Solid Edge part; units mm, degrees
sketch "Sketch1" plane through (0, 0, 0) normal (0, 0, 1) x (1, 0, 0)
  circle A0 centre (0, 0) radius 1.5
extrude "Protrusion1" add sketch "Sketch1" along normal blind 30
chamfer "Chaflán_1" distance 0.6 angle 45 1 edges at (-1.5, 0, 0)
sketch "Sketch2" plane through (0, 0, 30) normal (0, 0, 1) x (1, 0, 0)
  circle A0 centre (0, 0) radius 2.7
extrude "ProtrusiónExtruida_3" add sketch "Sketch2" along normal blind 2
sketch "Sketch3" plane through (0, 0, 32) normal (0, 0, 1) x (0, 1, 0)
  line L0 (0.5, -3.2084) -> (-0.5, -3.2084)
  line L1 (-0.5, -3.2084) -> (-0.5, 3.2084)
  line L2 (-0.5, 3.2084) -> (0.5, 3.2084)
  line L3 (0.5, 3.2084) -> (0.5, -3.2084)
extrude "VaciadoExtruido_5" cut sketch "Sketch3" against normal blind 1.148
properties material "Acero inoxidable, 303"
Here's how the part is built. I have some questions about the finished solid (model axes, mm). A direction names the side the tool comes from. Coordinates: 2 decimals unless noted, no trailing zeros. Order: outer loops, then holes, each group sorted by start corner. A loop starts at its lowest first (then second) coordinate and runs counter-clockwise, first axis right, second up.
1) I need wall thicknesses on line 1 (Y direction, x = -1.2, z = 21.5); line 2 (Z direction, x = 1.1, y = -1.25); line 3 (X direction, y = -0.55, z = 23). Which ranges of each line are inside material? Lowest first, please.
2) Imagine slicing it at B-B on x = 0. List the corners of the cut face in (y, z) for me.
3) We'd pull the mould along Y, two halves only. Please class faces 4 (the face through (1.2, -1.2, 30)), 5 (the face through (2.575, -0.811, 30.986)), 6 (the face through (0, 0.5, 31.4)): +Y half, -Y half, draft (parallel to the pull), parting line (faces both ways), or undercut.
4) Imagine slicing it at D-D on x = -2.3. List the corners of the cut face in (y, z) for me.
5) Imagine slicing it at A-A on y = 0. List the corners of the cut face in (x, z) for me.
6) Imagine slicing it at C-C on z = 6. List the corners of the cut face in (x, y) for me, and give its area (3 significant figures).
7) Will these pins go through, and if not, where does the flat tip stop? pin 1 (1 mm diameter, centred on x = -1, z = 10.5, fed in from -Y); pin 2 (1.5 mm diameter, centred on x = -1, z = 4.5, fed in from -Y); pin 3 (1 mm diameter, centred on x = -1, z = 15.5, fed in from +Y).
8) Which directions (+Z, -Z, +X, -X, +Y, -Y) give clear straight access to the entire face, cutting with the end or side of a thin tool? Please do faces 1 (the face through (0, -0.5, 31.4)), 2 (the face through (-1.5, -0.07, 15.09)), 3 (the face through (0, -1, 32)).
Response values:
1. line 1: y = -0.9 to 0.9
1. line 2: z = 30 to 32
1. line 3: x = -1.4 to 1.4
2. outline: (-2.7, 30) - (-1.5, 30) - (-1.5, 0.6) - (-0.9, 0) - (0.9, 0) - (1.5, 0.6) - (1.5, 30) - (2.7, 30) - (2.7, 32) - (0.5, 32) - (0.5, 30.85) - (-0.5, 30.85) - (-0.5, 32) - (-2.7, 32) - close
3. face 4: draft
3. face 5: parting line
3. face 6: undercut
4. outline: (-1.41, 30) - (1.41, 30) - (1.41, 32) - (0.5, 32) - (0.5, 30.85) - (-0.5, 30.85) - (-0.5, 32) - (-1.41, 32) - close
5. outline: (-2.7, 30) - (-1.5, 30) - (-1.5, 0.6) - (-0.9, 0) - (0.9, 0) - (1.5, 0.6) - (1.5, 30) - (2.7, 30) - (2.7, 30.85) - (-2.7, 30.85) - close
6. outline: circle Ø3 at (0, 0)
6. area: 7.07 mm2
7. pin 1: stops at y = -1.41
7. pin 2: stops at y = -1.48
7. pin 3: stops at y = 1.41
8. face 1: +Z, +X, -X
8. face 2: -Z
8. face 3: +Z, +X, -X, +Y, -Y
